Could you check a few things on this drawing? It's one solid part, dimensions in mm from its lowest x, y, z. A direction names the side the tool comes from. Round coordinates to 2 decimals unless told otherwise and drop trailing zeros. Loops run counter-clockwise (first coordinate to the right, second up) from the corner with the lowest first, then second, coordinate; pieces in that order, holes last.
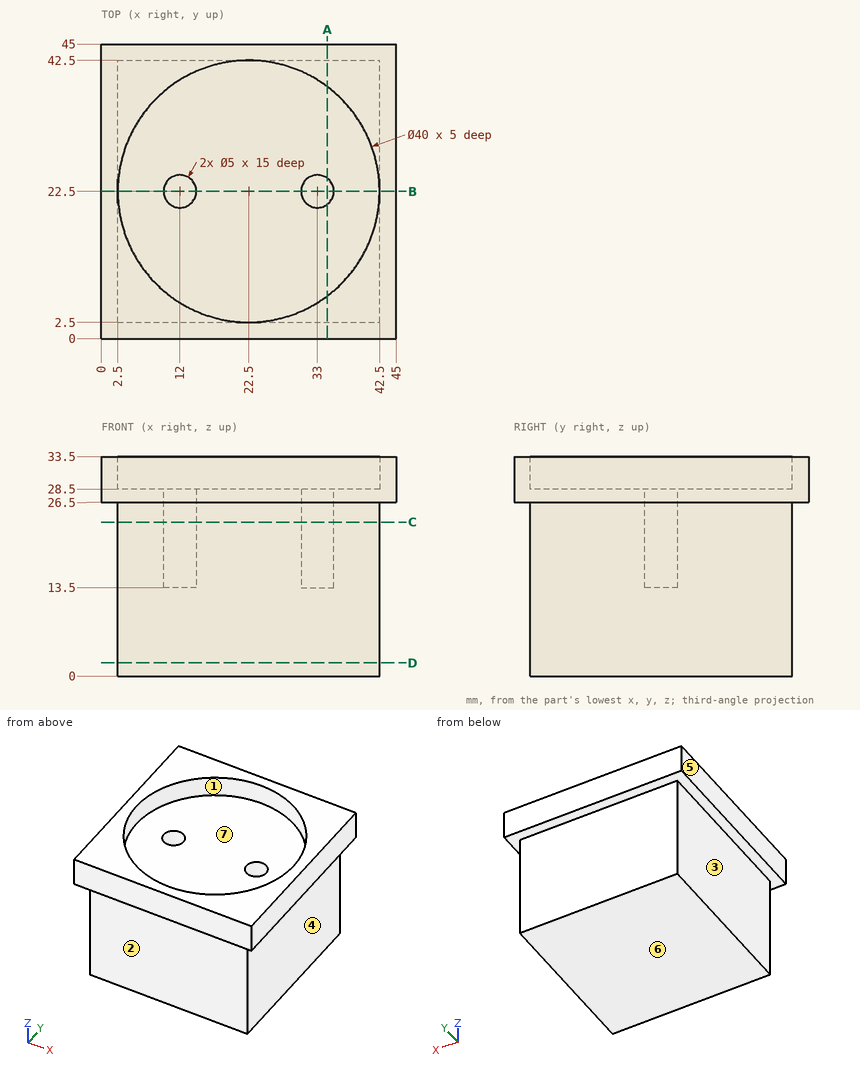
(1) Suppose I cut it at D-D (z = 2). Write out the boundary of the cut face in (x, y), then the cut area to 3 significant figures.
(2) Suppose I cut it at A-A (x = 34.5). Write out the boundary of the cut face in (y, z).
(3) For pin 1 (4 mm diameter, centred on x = 32, y = 22, fed in from +Z); pin 2 (8 mm diameter, centred on x = 17, z = 6, fed in from -Y); pin 3 (13.5 mm diameter, centred on x = 24, y = 19.5, fed in from -Z); pin 4 (4.5 mm diameter, centred on x = 33, y = 22.5, fed in from +Z), each with a flat end and sliding along its axis, tell me the tip position at first contact or that it passes through.
(4) Which directions (+Z, -Z, +X, -X, +Y, -Y) give clear straight access to the entire face, cutting with the end or side of a thin tool? Please do the marked faces 1, 2, 3 and 4.
(5) Suppose I cut it at C-C (z = 23.5). Write out the boundary of the cut face in (x, y).
(6) If I drill on line 1 (Y direction, x = 12, z = 18); line 2 (X direction, y = 22, z = 18); line 3 (Y direction, x = 22.5, z = 32), over which ranges is the centre line in solid material (lowest first)?
(7) Suppose I cut it at B-B (y = 22.5). Write out the boundary of the cut face in (x, z), then the cut area to 4 significant figures.
(8) We'd pull the mould along X, two halves only. Please class the marked faces 5, 6 and 7: released by +X, released by -X, zero draft, split by the parting line, or undercut.
Check result:
1. outline: (2.5, 2.5) - (42.5, 2.5) - (42.5, 42.5) - (2.5, 42.5) - close
1. area: 1,600 mm2
2. outline: (0, 26.5) - (2.5, 26.5) - (2.5, 0) - (42.5, 0) - (42.5, 26.5) - (45, 26.5) - (45, 33.5) - (38.5, 33.5) - (38.5, 28.5) - (24.5, 28.5) - (24.5, 13.5) - (20.5, 13.5) - (20.5, 28.5) - (6.5, 28.5) - (6.5, 33.5) - (0, 33.5) - close
3. pin 1: stops at z = 28.5
3. pin 2: stops at y = 2.5
3. pin 3: stops at z = 0
3. pin 4: stops at z = 13.5
4. face 1: +Z
4. face 2: -Z, +X, -X, -Y
4. face 3: -Z, -X, +Y, -Y
4. face 4: -Z, +X, +Y, -Y
5. outline: (2.5, 2.5) - (42.5, 2.5) - (42.5, 42.5) - (2.5, 42.5) - close; hole circle Ø5 at (12, 22.5); hole circle Ø5 at (33, 22.5)
6. line 1: y = 2.5 to 20, 25 to 42.5
6. line 2: x = 2.5 to 9.55, 14.45 to 30.55, 35.45 to 42.5
6. line 3: y = 0 to 2.5, 42.5 to 45
7. outline: (0, 26.5) - (2.5, 26.5) - (2.5, 0) - (42.5, 0) - (42.5, 26.5) - (45, 26.5) - (45, 33.5) - (42.5, 33.5) - (42.5, 28.5) - (35.5, 28.5) - (35.5, 13.5) - (30.5, 13.5) - (30.5, 28.5) - (14.5, 28.5) - (14.5, 13.5) - (9.5, 13.5) - (9.5, 28.5) - (2.5, 28.5) - (2.5, 33.5) - (0, 33.5) - close
7. area: 1,025 mm2
8. face 5: released by -X
8. face 6: zero draft
8. face 7: undercut
